Solid Edge part; units mm, degrees
sketch "Sketch1" plane through (0, 0, 0) normal (0, 0, 1) x (1, 0, 0)
  line L0 (-26.3559, 16.3207) -> (0, 16.3207)
  line L1 (0, 16.3207) -> (0, -16.3207)
  line L2 (0, -16.3207) -> (-26.3559, -16.3207)
  line L3 (-26.3559, -16.3207) -> (-26.3559, 16.3207)
extrude "Protrusion1" add sketch "Sketch1" along normal up to vertex (7.5 mm away)
sketch "Sketch2" plane through (0.0003, -13.7602, 7.5) normal (0, 0, 1) x (-1, 0, 0)
  circle A0 centre (8.5228, -5.2346) radius 1.7
  circle A1 centre (8.5231, -22.2805) radius 1.7
extrude "Cutout1" cut sketch "Sketch2" against normal up to next
sketch "Sketch3" plane through (0.0003, -13.7602, 7.5) normal (0, 0, 1) x (0, 1, 0)
  circle A0 centre (5.2346, 8.5228) radius 2.5
  circle A1 centre (22.2805, 8.5231) radius 2.5
extrude "Cutout2" cut sketch "Sketch3" against normal blind 5
sketch "Sketch4" plane through (0, 0, 3.5) normal (1, 0, 0) x (0, 1, 0)
  line L0 (-16.3207, 4) -> (16.3207, 4)
  line L1 (16.3207, 4) -> (16.3207, 3.5)
  arc A0 (-16.3207, 3.5) -> (16.3207, 3.5) centre (0, 34.9133) ccw
  line L2 (-16.3207, 4) -> (-16.3207, 3.5)
extrude "Cutout3" cut sketch "Sketch4" against normal blind 24.9
sketch "Sketch5" plane through (0, 0, 3.5) normal (1, 0, 0) x (0, 1, 0)
  circle A0 centre (-13.3207, 0) radius 1.5
  circle A1 centre (13.3207, 0) radius 1.531
extrude "Protrusion2" add sketch "Sketch5" along normal blind 7
sketch "Sketch6" plane through (-26.3559, -27.5204, 3.5) normal (-1, 0, 0) x (0, 0, 1)
  line L0 (4, 43.8411) -> (18, 41.3725)
  arc A0 (18, 41.3725) -> (18, 13.6682) centre (34.1805, 27.5204) cw
  line L1 (4, 11.1997) -> (18, 13.6682)
  line L2 (-3.5, 11.1997) -> (4, 11.1997)
  line L3 (-3.5, 43.8411) -> (-3.5, 11.1997)
  line L4 (4, 43.8411) -> (-3.5, 43.8411)
extrude "Protrusion3" add sketch "Sketch6" against normal up to vertex (1.4559 mm away)
sketch "Sketch7" plane through (-26.3559, -27.5204, 30.1014) normal (-1, 0, 0) x (0, -1, 0)
  circle A0 centre (-17.2704, -0.7209) radius 1.15
  circle A1 centre (-17.2704, -21.4209) radius 1.15
  circle A2 centre (-37.7704, -21.4209) radius 1.15
  circle A3 centre (-37.7704, -0.7209) radius 1.15
  arc A4 (-35.1204, -0.6522) -> (-19.9204, -0.6522) centre (-27.5204, 7.5791) cw
  line L0 (-19.9204, -0.6522) -> (-19.9204, -27.819)
  line L1 (-19.9204, -27.819) -> (-35.1204, -27.819)
  line L2 (-35.1204, -27.819) -> (-35.1204, -0.6522)
extrude "Cutout4" cut sketch "Sketch7" against normal up to next
For this review, take the finished solid that the model builds, in its own axes (mm). A direction names the side the tool comes from. Coordinates: 2 decimals unless noted, no trailing zeros. Order: outer loops, then holes, each group sorted by start corner. A loop starts at its lowest first (then second) coordinate and runs counter-clockwise, first axis right, second up. Notation, with made-up numbers: (-29, 5.5) -> (-8, 5.5) arc R14 cw to (-8, 19.5) -> close; hole circle Ø7 at (-24, -32.75). An arc over 180 degrees is marked (long way). Use CSV: the item, a comma, the result in double quotes. Start each with the question number.
Item 1: Wall thickness on probe 1 along Z at (x, y) = (-11, 3.5); probe 2 along Z at (x, y) = (-25.6, 10.25); probe 3 along X at (y, z) = (-10, 6): over which ranges is each line inside the solid? List them lowest first.
Item 2: Draft analysis for pull direction Z (two halves, no side actions). For faces 1 (the face through (-25.638, 9.188, 8.24)), 2 (the face through (-12.276, -12.126, 5.155)), 3 (the face through (7, -13, 3)), 4 (the face through (-25.638, 15.104, 14.402)), state which applies: pulls with the +Z half, pulls with the -Z half, needs draft (parallel to the pull), parting line crosses it, or undercut.
Item 3: For faces 5 (the face through (-12.28, 12, 5.11)), 6 (the face through (-8.591, -11.025, 3.401)), 7 (the face through (-25.638, 9.153, 29.726)), 8 (the face through (-25.638, -15.104, 14.402)), 9 (the face through (0, 0, 2)), list the 3-axis set-ups (+Z, -Z, +X, -X, +Y, -Y) from which the entire face can be reached by the end or side of a thin tool; tool diameter is ignored.
Item 4: We need section D-D, the plane x = -8. Give the boundary of the cut face in (y, z), then the cut area to 3 significant figures.
Item 5: Insertion check: pin 1 (21.5 mm diameter, centred on y = 6, z = 29.5, fed in from +X); pin 2 (0.5 mm diameter, centred on x = -4.5, z = 3, fed in from -Y); pin 3 (16.5 mm diameter, centred on x = -10, y = -0.5, fed in from +Z); pin 4 (2 mm diameter, centred on x = -22.5, y = 1.5, fed in from -Z). Each pin has a flat end and moves straight along its axis. Give the tip position at first contact, or say it passes through.
Item 6: We need section A-A, the plane y = 0. Give the boundary of the cut face in (x, z).
Item 7: We need section B-B, the plane x = 2.5. Give the boundary of the cut face in (y, z).
Item 8: We need section C-C, the plane z = 34. Give the boundary of the cut face in (x, y).
Derived:
1,probe 1,"z = 0 to 2.28"
1,probe 2,"z = 0 to 7.53, 9.83 to 28.23, 30.53 to 33.16, 42.2 to 56.35"
1,probe 3,"x = -26.36 to -24.9"
2,face 1,"undercut"
2,face 2,"pulls with the +Z half"
2,face 3,"needs draft"
2,face 4,"undercut"
3,face 5,"+Z, +X"
3,face 6,"+Z"
3,face 7,"+X, -X"
3,face 8,"+X, -X, -Y"
3,face 9,"+X"
4,outline,"(-16.32, 0) -> (-10.14, 0) -> (-10.14, 2.5) -> (-10.97, 2.5) -> (-10.97, 4.76) arc R35.4 cw to (-16.32, 7) -> close; (-6.91, 0) -> (6.9, 0) -> (6.9, 2.28) -> (-6.91, 2.28) -> close; (10.14, 0) -> (16.32, 0) -> (16.32, 7) arc R35.4 cw to (10.97, 4.75) -> (10.97, 2.5) -> (10.14, 2.5) -> close"
4,area,"97.7 mm^2"
5,pin 1,"stops at x = -24.9"
5,pin 2,"stops at y = -16.32"
5,pin 3,"stops at z = 4.1"
5,pin 4,"stops at z = 0"
6,outline,"(-26.36, 0) -> (0, 0) -> (0, 2.28) -> (-26.36, 2.28) -> close; (-26.36, 48.88) -> (-24.9, 48.88) -> (-24.9, 58.98) -> (-26.36, 58.98) -> close"
7,outline,"circle Ø3 at (-13.32, 3.5); circle Ø3.06 at (13.32, 3.5)"
8,outline,"(-26.36, -20.98) -> (-24.9, -20.98) -> (-24.9, -10.58) -> (-26.36, -10.58) -> close; (-26.36, 10.58) -> (-24.9, 10.58) -> (-24.9, 20.98) -> (-26.36, 20.98) -> close"
